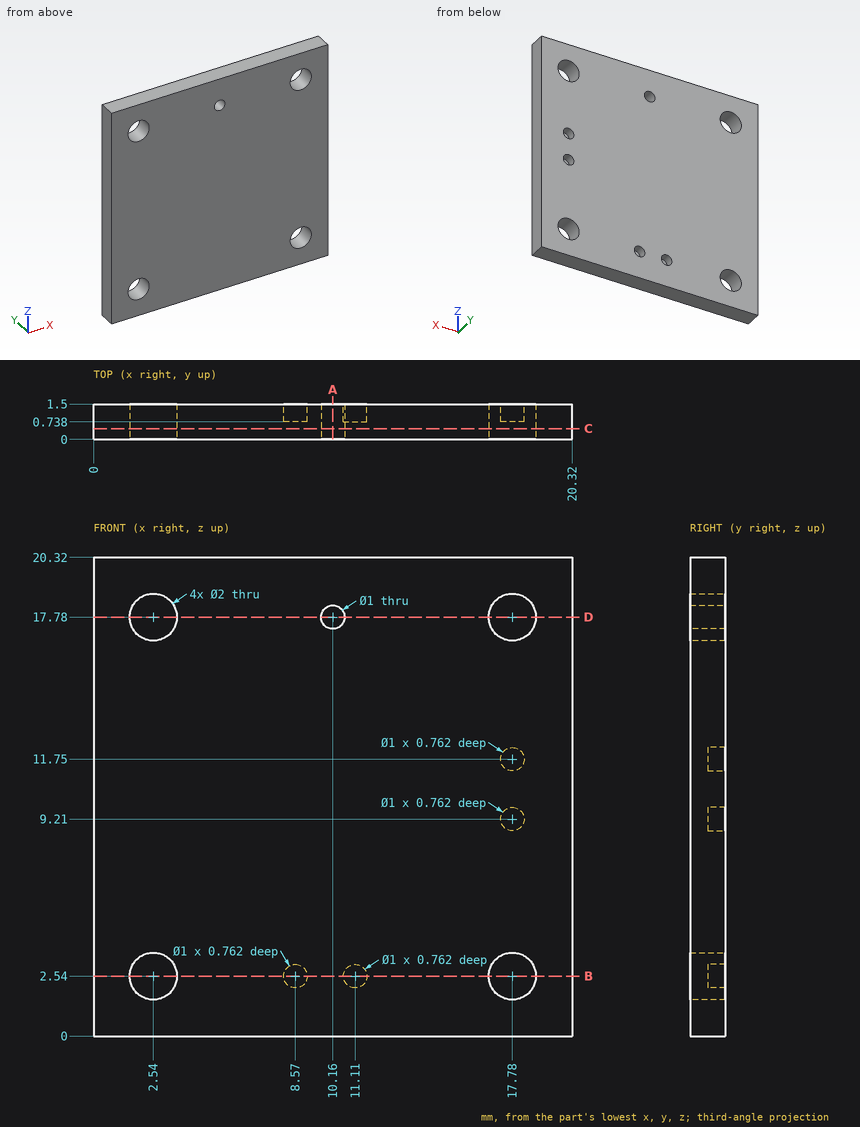
The drawing under review shows one solid part. Ordinate dimensions are in mm from its lowest x, y, z. Round coordinates to 2 decimals unless told otherwise and drop trailing zeros. Loops run counter-clockwise (first coordinate to the right, second up) from the corner with the lowest first, then second, coordinate; pieces in that order, holes last. Notation, with made-up numbers: (44.5, -23.5) - (101.5, -23.5) arc R23 cw to (101.5, 11.5) - close; hole circle Ø9 at (83, 0.25). An arc over 180 degrees is marked (long way). Put each result on its own line as item: value. Start each with the question number.
1. For probe 1 along X at (y, z) = (0.6, 2.54); probe 2 along X at (y, z) = (1.1, 17.78); probe 3 along X at (y, z) = (1.1, 2.54), list the stretches that pass through material, from the lowest coordinate up. Write a range as [from, to].
2. Consider section D-D on z = 17.78. State the section outline as (x, y) points.
3. Consider section A-A on x = 10.16. State the section outline as (y, z) points.
4. Consider section C-C on y = 0.45. State the section outline as (x, z) points, plus the area to 3 significant figures.
5. Consider section B-B on z = 2.54. State the section outline as (x, y) points.
6. Insertion check: P1, Ø0.5, axis at x = 11, z = 2.5, coming from the +Y side; P2, Ø1.6, axis at x = 17.78, z = 2.54, coming from the +Y side. Each pin has a flat end and moves straight along its axis. Give the tip position at first contact, or say it passes through.
Result sheet:
1. probe 1: [0, 1.54], [3.54, 16.78], [18.78, 20.32]
1. probe 2: [0, 1.54], [3.54, 9.66], [10.66, 16.78], [18.78, 20.32]
1. probe 3: [0, 1.54], [3.54, 8.07], [9.07, 10.61], [11.61, 16.78], [18.78, 20.32]
2. outline: (0, 0) - (1.54, 0) - (1.54, 1.5) - (0, 1.5) - close; (3.54, 0) - (9.66, 0) - (9.66, 1.5) - (3.54, 1.5) - close; (10.66, 0) - (16.78, 0) - (16.78, 1.5) - (10.66, 1.5) - close; (18.78, 0) - (20.32, 0) - (20.32, 1.5) - (18.78, 1.5) - close
3. outline: (0, 0) - (1.5, 0) - (1.5, 17.28) - (0, 17.28) - close; (0, 18.28) - (1.5, 18.28) - (1.5, 20.32) - (0, 20.32) - close
4. outline: (0, 0) - (20.32, 0) - (20.32, 20.32) - (0, 20.32) - close; hole circle Ø2 at (2.54, 2.54); hole circle Ø2 at (2.54, 17.78); hole circle Ø1 at (10.16, 17.78); hole circle Ø2 at (17.78, 2.54); hole circle Ø2 at (17.78, 17.78)
4. area: 400 mm^2
5. outline: (0, 0) - (1.54, 0) - (1.54, 1.5) - (0, 1.5) - close; (3.54, 0) - (16.78, 0) - (16.78, 1.5) - (11.61, 1.5) - (11.61, 0.74) - (10.61, 0.74) - (10.61, 1.5) - (9.07, 1.5) - (9.07, 0.74) - (8.07, 0.74) - (8.07, 1.5) - (3.54, 1.5) - close; (18.78, 0) - (20.32, 0) - (20.32, 1.5) - (18.78, 1.5) - close
6. P1: y = 0.74
6. P2: through
